Work out the finished part from the listing and answer in its coordinate system (mm). A direction names the side the tool comes from. Coordinates: 2 decimals unless noted, no trailing zeros. Order: outer loops, then holes, each group sorted by start corner. A loop starts at its lowest first (then second) coordinate and runs counter-clockwise, first axis right, second up.
```python
from build123d import *

# Parameters (mm, degrees)
SKETCH_1_W          = 19
SKETCH_1_H          = 40
EXTRUDE_1_DEPTH     = 1.6
FILLET_1_R          = 2
CUT_EXTRUDE_1_DEPTH = 45.312075104


with BuildPart() as part:
    # Эскиз1 → Бобышка-Вытянуть1 (new body)
    with BuildSketch(Plane.XY):
        with Locations((9.5, 20)):
            Rectangle(SKETCH_1_W, SKETCH_1_H)
    extrude(amount=EXTRUDE_1_DEPTH)

    # Скругление1
    fillet_1_edges = [part.edges().sort_by_distance(p)[0] for p in [
        (0, 40, 0.8),
        (19, 40, 0.8),
        (19, 0, 0.8),
        (0, 0, 0.8),
    ]]
    fillet(fillet_1_edges, radius=FILLET_1_R)

    # Эскиз3 → Вырез-Вытянуть1 (cut, through all)
    with BuildSketch(Plane.XY.offset(1.6)):
        with BuildLine():
            Line((15.1, 2.893381891), (15.1, 9.893381891))
            ThreePointArc((15.1, 9.893381891), (16.2, 10.993381891), (17.3, 9.893381891))
            Line((17.3, 9.893381891), (17.3, 2.893381891))
            ThreePointArc((17.3, 2.893381891), (16.2, 1.793381891), (15.1, 2.893381891))
        make_face()
        with BuildLine():
            Line((15.1, 30.893381891), (15.1, 37.893381891))
            ThreePointArc((15.1, 37.893381891), (16.2, 38.993381891), (17.3, 37.893381891))
            Line((17.3, 37.893381891), (17.3, 30.893381891))
            ThreePointArc((17.3, 30.893381891), (16.2, 29.793381891), (15.1, 30.893381891))
        make_face()
    extrude(amount=-CUT_EXTRUDE_1_DEPTH, mode=Mode.SUBTRACT)


solid = part.part
```
1. A flat-ended cylindrical pin translates along its axis: pin 1 (2 mm diameter, centred on x = 8.5, y = 18.5, fed in from -Z). Find the tip coordinate at first contact, or state that the pin passes through.
2. The part is cut by section C-C (x = 16.2). Determine the outline of the cut face in (y, z).
3. For faces 5 (the flat face through (9, 20, 0)), 6 (the flat face through (15.1, 34, 1)), determine the directions among +Z, -Z, +X, -X, +Y, -Y from which every point of the face is accessible in a straight line to the end or side of a thin tool.
4. The part is cut by section A-A (y = 8). Determine the outline of the cut face in (x, z), plus the area to 3 significant figures.
5. The mould has two halves that part along X. Classify faces 1 (the cylindrical face through (18.4, 0.57, 0.81)), 2 (the flat face through (9, 40, 1)), 3 (the flat face through (0, 20, 1)), 4 (the cylindrical face through (16.224, 1.794, 0.811)): released by +X, released by -X, zero draft, split by the parting line, or undercut.
6. The part is cut by section B-B (z = 1). Determine the outline of the cut face in (x, y), plus the area to 3 significant figures.
7. Consider probe 1 along X at (y, z) = (5, 1.2); probe 2 along Y at (x, z) = (18.25, 1.05). Determine where each line is inside the solid, lowest interval first.
Worked out:
1. pin 1: stops at z = 0
2. outline: (0, 0) - (1.79, 0) - (1.79, 1.6) - (0, 1.6) - close; (10.99, 0) - (29.79, 0) - (29.79, 1.6) - (10.99, 1.6) - close; (38.99, 0) - (40, 0) - (40, 1.6) - (38.99, 1.6) - close
3. face 5: -Z, +X, -X, +Y, -Y
3. face 6: +Z, -Z
4. outline: (0, 0) - (15.1, 0) - (15.1, 1.6) - (0, 1.6) - close; (17.3, 0) - (19, 0) - (19, 1.6) - (17.3, 1.6) - close
4. area: 26.9 mm2
5. face 1: released by +X
5. face 2: zero draft
5. face 3: released by -X
5. face 4: undercut
6. outline: (0, 2) arc R2 ccw to (2, 0) - (17, 0) arc R2 ccw to (19, 2) - (19, 38) arc R2 ccw to (17, 40) - (2, 40) arc R2 ccw to (0, 38) - close; hole (15.1, 2.89) arc R1.1 ccw to (17.3, 2.89) - (17.3, 9.89) arc R1.1 ccw to (15.1, 9.89) - close; hole (15.1, 30.89) arc R1.1 ccw to (17.3, 30.89) - (17.3, 37.89) arc R1.1 ccw to (15.1, 37.89) - close
6. area: 718 mm2
7. probe 1: x = 0 to 15.1, 17.3 to 19
7. probe 2: y = 0.44 to 39.56
